```python
from build123d import *

# Parameters (mm, degrees)
F0_R     = 2.5
F0_R_2   = 1.25
F1_DEPTH = 10
F2_R     = 2
F4_D     = 2.5
F4_DEPTH = 4.5
F4_TIP   = 0.7510757738


with BuildPart() as f1:
    # F0 (on Top) → F1 (new body)
    with BuildSketch(Plane.XY):
        Circle(F0_R)
        Circle(F0_R_2, mode=Mode.SUBTRACT)
        Circle(F0_R_2)
    extrude(amount=F1_DEPTH)

    # F2
    f2_edges = [f1.edges().sort_by_distance(p)[0] for p in [
        (-2.5, 0, 10),
    ]]
    fillet(f2_edges, radius=F2_R)

    # F4
    with Locations(Plane(origin=(0, 0, 0), x_dir=(1, 0, 0), z_dir=(0, 0, -1))):
        with Locations((0, 0)):
            Hole(F4_D / 2, depth=F4_DEPTH)
            with Locations((0, 0, -(F4_DEPTH + F4_TIP / 2))):  # 118° drill point
                Cone(0, F4_D / 2, F4_TIP, mode=Mode.SUBTRACT)


solid = f1.part
```
Read the model definition and answer for the solid it produces. Units are mm, in the model's axes. Give positions to 0.01 mm unless a question says otherwise; leave off trailing zeros. Order: outer loops, then holes, each group sorted by start corner. A loop starts at its lowest first (then second) coordinate and runs counter-clockwise, first axis right, second up.
(1) Straight lines are drawn through the part: L1, parallel to Y at x = 0, z = 3.3; L2, parallel to X at y = 0.3, z = 1.5; L3, parallel to Y at x = 0.95, z = 1.75. For each, find the intervals that lie inside material, in ascending order.
(2) Find section A-A (z = 6.25). Give the vertices of the cut face in (x, y).
(3) For a pull along X with two mould halves and no side action, classify faces 1 (the cylindrical face through (0.27, 1.22, 2.28)), 2 (the flat face through (-1, -1, 0)), 3 (the cylindrical face through (-0.54, -2.44, 3.94)) as released by +X, released by -X, zero draft, split by the parting line, or undercut.
(4) Given pin 1 (1 mm diameter, centred on x = -1.5, z = 1.5, fed in from -Y); pin 2 (1.5 mm diameter, centred on y = -1.5, z = 7.5, fed in from +X); pin 3 (1.5 mm diameter, centred on x = 1.5, y = 0.5, fed in from +Z), each flat-ended and moving along its own axis, determine where each tip first touches the part or whether it passes through.
Result sheet:
1. L1: y = -2.5 to -1.25, 1.25 to 2.5
1. L2: x = -2.48 to -1.21, 1.21 to 2.48
1. L3: y = -2.31 to -0.81, 0.81 to 2.31
2. outline: circle Ø5 at (0, 0)
3. face 1: undercut
3. face 2: zero draft
3. face 3: split by the parting line
4. pin 1: stops at y = -2.29
4. pin 2: stops at x = 2.38
4. pin 3: stops at z = 9.97
